The listing builds one solid part. Answer for the finished solid, in the listing's coordinates (mm). A direction names the side the tool comes from. Give positions to 0.01 mm unless a question says otherwise; leave off trailing zeros. Write each loop counter-clockwise with the first axis right and the second up, starting at its lowest first coordinate (ties: lowest second). Pieces come first, ordered by that corner, then holes. Notation, with made-up numbers: (17, -31) -> (33, -31) arc R31 cw to (33, -5) -> close; hole circle Ø9 at (-24, 23). An arc over 180 degrees is marked (long way). One line per question, with ' | ' between items.
from build123d import *

# Parameters (mm, degrees)
SKETCH1_W                = 84
SKETCH1_H                = 42
SKETCH1_R                = 1.4
BOSS_EXTRUDE1_DEPTH      = 3
BOSS_EXTRUDE2_DEPTH      = 20
BOSS_EXTRUDE2_DEPTH_BACK = 3
SKETCH2_W                = 84
SKETCH2_H                = 3
FILLET1_R                = 3
SKETCH5_R                = 2.75
CUT_EXTRUDE1_DEPTH       = 3


with BuildPart() as part:
    # Sketch1 → Boss-Extrude1 (new body)
    with BuildSketch(Plane.XY):
        Rectangle(SKETCH1_W, SKETCH1_H)
        with Locations((-37.7, 15.7)):
            Circle(SKETCH1_R, mode=Mode.SUBTRACT)
        with Locations((37.7, 15.7)):
            Circle(SKETCH1_R, mode=Mode.SUBTRACT)
        with Locations((37.7, -15.7)):
            Circle(SKETCH1_R, mode=Mode.SUBTRACT)
        with Locations((-37.7, -15.7)):
            Circle(SKETCH1_R, mode=Mode.SUBTRACT)
    extrude(amount=BOSS_EXTRUDE1_DEPTH)

    # Sketch2 → Boss-Extrude2 (add, two sides: drawn at the far end of the back side and taken through both)
    with BuildSketch(Plane(origin=(0, 0, 0), x_dir=(-1, 0, 0), z_dir=(0, 0, -1)).offset(-BOSS_EXTRUDE2_DEPTH_BACK)):
        with Locations((0, -22.5)):
            Rectangle(SKETCH2_W, SKETCH2_H)
    extrude(amount=BOSS_EXTRUDE2_DEPTH + BOSS_EXTRUDE2_DEPTH_BACK)

    # Fillet1
    fillet1_edges = [part.edges().sort_by_distance(p)[0] for p in [
        (0, -21, 0),
    ]]
    fillet(fillet1_edges, radius=FILLET1_R)

    # Sketch5 → Cut-Extrude1 (cut)
    with BuildSketch(Plane(origin=(0, -21, 0), x_dir=(1, 0, 0), z_dir=(0, 1, 0))):
        with Locations(Location((-32, 11.5, 0), (0, 0, 270))):
            Circle(SKETCH5_R)
        with Locations(Location((32, 11.5, 0), (0, 0, 270))):
            Circle(SKETCH5_R)
    extrude(amount=-CUT_EXTRUDE1_DEPTH, mode=Mode.SUBTRACT)


solid = part.part
Item 1: Find section B-B (x = -37.7). Write down the section's boundary in (y, z).
Answers below:
outline: (-24, -20) -> (-21, -20) -> (-21, -3) arc R3 cw to (-18, 0) -> (-17.1, 0) -> (-17.1, 3) -> (-24, 3) -> close; (-14.3, 0) -> (14.3, 0) -> (14.3, 3) -> (-14.3, 3) -> close; (17.1, 0) -> (21, 0) -> (21, 3) -> (17.1, 3) -> close
Item 2: Flat-ended cylindrical pins translate along their axes: pin 1 (3 mm diameter, centred on x = -3.5, y = -13, fed in from -Z); pin 2 (7 mm diameter, centred on x = 32, z = -11.5, fed in from +Y); pin 3 (2.5 mm diameter, centred on x = -37.7, y = -15.7, fed in from +Z). Find the tip coordinate at first contact, or state that the pin passes through.
Answers below:
pin 1: z = 0 | pin 2: y = -21 | pin 3: through
Item 3: A tool of negligible diameter and unlimited length cuts with its end or side. For faces 4 (the face through (-29.273, -22.479, -11.858)), 5 (the face through (-1, 2, 0)), from which of +Z, -Z, +X, -X, +Y, -Y can it reach the whole face along a straight path? Write none if from no direction.
Answers below:
face 4: +Y, -Y | face 5: -Z, +X, -X, +Y
Item 4: Determine the mould class of faces 1 (the face through (-42, -7, 1)), 2 (the face through (34.727, -22.479, -11.858)), 3 (the face through (1, -1, 3)) for opening direction Z: pulls with the +Z half, pulls with the -Z half, needs draft (parallel to the pull), parting line crosses it, or undercut.
Answers below:
face 1: needs draft | face 2: undercut | face 3: pulls with the +Z half
Item 5: Find section D-D (z = -4.25). Write down the section's boundary in (x, y).
Answers below:
outline: (-42, -24) -> (42, -24) -> (42, -21) -> (-42, -21) -> close
Item 6: Find section A-A (y = -15.7). Write down the section's boundary in (x, z).
Answers below:
outline: (-42, 0) -> (-39.1, 0) -> (-39.1, 3) -> (-42, 3) -> close; (-36.3, 0) -> (36.3, 0) -> (36.3, 3) -> (-36.3, 3) -> close; (39.1, 0) -> (42, 0) -> (42, 3) -> (39.1, 3) -> close
Item 7: Find section C-C (x = 26). Write down the section's boundary in (y, z).
Answers below:
outline: (-24, -20) -> (-21, -20) -> (-21, -3) arc R3 cw to (-18, 0) -> (21, 0) -> (21, 3) -> (-24, 3) -> close
Item 8: Consider line 1 (Y direction, x = 37.7, z = 0.65); line 2 (Z direction, x = 21, y = -5); line 3 (Y direction, x = -38, z = -4.75). Determine where each line is inside the solid, lowest interval first. Write a range as [from, to].
Answers below:
line 1: [-24, -17.1], [-14.3, 14.3], [17.1, 21] | line 2: [0, 3] | line 3: [-24, -21]
